Check sheet for the modelled part. Datum: model origin and axes. Units: mm. A direction names the side the tool comes from. Give positions to 0.01 mm unless a question says otherwise; leave off trailing zeros. Loops run counter-clockwise (first coordinate to the right, second up) from the corner with the lowest first, then second, coordinate; pieces in that order, holes last. Notation, with made-up numbers: (-8.5, -36.75) -> (18.5, -36.75) arc R27 cw to (18.5, -3.75) -> close; hole circle Ø7 at (17.25, 11.25). An arc over 180 degrees is marked (long way). Write each question's results on one line, items separated by ' | '. Start each with the question number.
Item 1: Scan lines: line 1 along Y through (x, z) = (38.5, -42); line 2 along X through (y, z) = (74.5, -90); line 3 along Z through (x, y) = (33, 27). Record each from-to range of solid material in increasing order.
Item 2: Access from +Z, -Z, +X, -X, +Y, -Y to the whole of each face (thin tool, end or side, straight path). Record for faces 1 (the face through (-78.067, -1581.683, 0.175)), 2 (the face through (55, -1552, 12.5)), 3 (the face through (104.74, -1556.817, 0.175)).
Item 3: Mould release check, pull along Y, two halves, no side actions. Record for faces 4 (the face through (55, -1552, -12.5)), 5 (the face through (1, 350, -1)), 6 (the face through (93.714, -1583.058, 0.175)): pulls with the +Y half, pulls with the -Y half, needs draft (parallel to the pull), parting line crosses it, or undercut.
Item 4: Cross-section at A-A on y = -1593. Enter the section's corners in (x, z), then the cut area to 3 significant figures.
Item 5: Cross-section at B-B on y = -1360.5. Enter the section's corners in (x, z).
Item 6: Gauge pin test, flat ends, axial feed: pin 1 Ø2.5 at (x, z) = (0.5, -14.5) entering from -Y; pin 2 Ø3 at (x, y) = (7.5, -1166) entering from -Z; pin 3 Ø17 at (x, z) = (162.5, -1.5) entering from +Y. Record the tip position at first contact, or that the pin passes through.
from build123d import *

# Parameters (mm, degrees)
CROQUIS1_R              = 100
SALIENTE_EXTRUIR1_DEPTH = 350
REDONDEO1_R             = 15
CROQUIS2_R              = 15.374662703
SALIENTE_EXTRUIR2_DEPTH = 1500
SALIENTE_EXTRUIR3_DEPTH = 12.5


with BuildPart() as part:
    # Croquis1 → Saliente-Extruir1 (new body)
    with BuildSketch(Plane(origin=(0, 0, 0), x_dir=(1, 0, 0), z_dir=(0, 1, 0))):
        with Locations(Location((0, 0, 0), (0, 0, 270))):
            Circle(CROQUIS1_R)
    extrude(amount=SALIENTE_EXTRUIR1_DEPTH)

    # Redondeo1
    redondeo1_edges = [part.edges().sort_by_distance(p)[0] for p in [
        (0, 0, -100),
        (0, 350, -100),
    ]]
    fillet(redondeo1_edges, radius=REDONDEO1_R)

    # Croquis2 → Saliente-Extruir2 (add)
    with BuildSketch(Plane.XZ):
        with Locations(Location((0, 0, 0), (0, 0, 90))):
            Circle(CROQUIS2_R)
    extrude(amount=SALIENTE_EXTRUIR2_DEPTH)

    # Croquis3 → Saliente-Extruir3 (add, symmetric)
    with BuildSketch(Plane.XY):
        Polygon((15.374662703, -1500), (196.643299481, -1615.247729776), (196.643299481, -1757.608907892), (169.890863325, -1757.608907892), (138.99299414, -1757.608907892), (119.105323431, -1707.327980329), (129.049158786, -1703.39488417), (154.441928733, -1743.657312209), (169.890863325, -1743.657312209), (169.890863325, -1631.4902803), (15.374662703, -1533.251325939), (-15.374662703, -1533.251325939), (-142.53937321, -1631.4902803), (-142.53937321, -1739.389775564), (-124.574455385, -1739.389775564), (-120.173982412, -1732.468444111), (-100.774753954, -1701.956158064), (-87.000489723, -1707.327980329), (-106.60953756, -1757.608907892), (-142.53937321, -1757.608907892), (-168.799765014, -1757.608907892), (-168.799765014, -1618.525977557), (-158.626316744, -1610.66665152), (-15.374662703, -1500), align=None)
    extrude(amount=SALIENTE_EXTRUIR3_DEPTH, both=True)


solid = part.part
Answer sheet:
1) line 1: y = 0 to 350 | line 2: x = -43.59 to 43.59 | line 3: z = -94.4 to 94.4
2) face 1: +Z, -Z | face 2: +Z, +X, -X, -Y | face 3: +Z, -Z, +X
3) face 4: needs draft | face 5: pulls with the +Y half | face 6: undercut
4) outline: (-135.76, -12.5) -> (-92.72, -12.5) -> (-92.72, 12.5) -> (-135.76, 12.5) -> close; (109.35, -12.5) -> (161.65, -12.5) -> (161.65, 12.5) -> (109.35, 12.5) -> close | area: 2,380 mm²
5) outline: circle Ø30.75 at (0, 0)
6) pin 1: stops at y = -1500 | pin 2: stops at z = -14.16 | pin 3: stops at y = -1588.14
